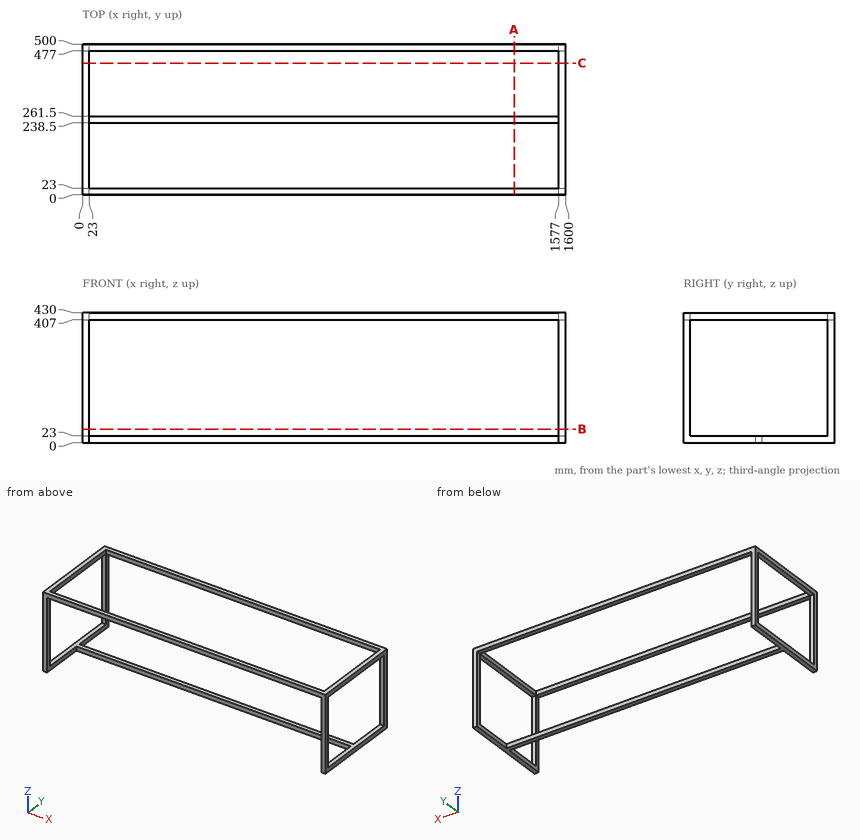
Geometry: see drawing. Coordinates: mm, zero at the bounding-box minimum. Give positions to 0.01 mm unless a question says otherwise; leave off trailing zeros. Loops run counter-clockwise (first coordinate to the right, second up) from the corner with the lowest first, then second, coordinate; pieces in that order, holes last. Notation, with made-up numbers: (-12, 25) - (35, 25) arc R18 cw to (35, 41) - close; hole circle Ø6 at (1.25, 76.25). An arc over 180 degrees is marked (long way). Use CSV: the item, a comma, the result in double quotes.
1) Cut plane B-B (z = 45). Output: boundary loops of the cut face in (x, y), and give its area (3 significant figures).
Worked out:
outline,"(0, 0) - (23, 0) - (23, 23) - (0, 23) - close; (0, 477) - (23, 477) - (23, 500) - (0, 500) - close; (1577, 0) - (1600, 0) - (1600, 23) - (1577, 23) - close; (1577, 477) - (1600, 477) - (1600, 500) - (1577, 500) - close"
area,"2,120 mm^2"
2) Cut plane A-A (x = 1429.5). Output: boundary loops of the cut face in (y, z), and give its area (3 significant figures).
Worked out:
outline,"(0, 407) - (23, 407) - (23, 430) - (0, 430) - close; (238.5, 0) - (261.5, 0) - (261.5, 23) - (238.5, 23) - close; (477, 407) - (500, 407) - (500, 430) - (477, 430) - close"
area,"1,590 mm^2"
3) Pin query (flat end, axial travel): P1, Ø11.5, axis at y = 325, z = 415, coming from the -X side; P2, Ø18.5, axis at x = 1030.5, z = 11.5, coming from the -Y side. Return the tip coordinate at first contact, or that it passes through.
Worked out:
P1,"stops at x = 0"
P2,"stops at y = 238.5"
4) Line query: line 1 (X direction, y = 208.5, z = 21.5); line 2 (Z direction, x = 1001, y = 253). Output: solid intervals per line, ascending.
Worked out:
line 1,"x = 0 to 23, 1577 to 1600"
line 2,"z = 0 to 23"
5) Cut plane C-C (y = 437). Output: boundary loops of the cut face in (x, z), and give its area (3 significant figures).
Worked out:
outline,"(0, 0) - (23, 0) - (23, 23) - (0, 23) - close; (0, 407) - (23, 407) - (23, 430) - (0, 430) - close; (1577, 0) - (1600, 0) - (1600, 23) - (1577, 23) - close; (1577, 407) - (1600, 407) - (1600, 430) - (1577, 430) - close"
area,"2,120 mm^2"
